from build123d import *

# Parameters (mm, degrees)
SKETCH1_R                = 40
SKETCH1_R_2              = 2.25
BOSS_EXTRUDE1_DEPTH      = 5
SKETCH2_R                = 30
SKETCH2_R_2              = 10
SKETCH2_R_3              = 2.5
BOSS_EXTRUDE2_DEPTH      = 5.5
BOSS_EXTRUDE2_DEPTH_BACK = 10.5
SKETCH3_R                = 2.5
SKETCH3_R_2              = 10
CUT_EXTRUDE1_DEPTH       = 17


with BuildPart() as part:
    # Sketch1 → Boss-Extrude1 (new body)
    with BuildSketch(Plane(origin=(0, 0, 0), x_dir=(1, 0, 0), z_dir=(0, 1, 0))):
        Circle(SKETCH1_R)
        with Locations((0, 35)):
            Circle(SKETCH1_R_2, mode=Mode.SUBTRACT)
        with Locations((30.310889132, 17.5)):
            Circle(SKETCH1_R_2, mode=Mode.SUBTRACT)
        with Locations((30.310889132, -17.5)):
            Circle(SKETCH1_R_2, mode=Mode.SUBTRACT)
        with Locations((0, -35)):
            Circle(SKETCH1_R_2, mode=Mode.SUBTRACT)
        with Locations((-30.310889132, -17.5)):
            Circle(SKETCH1_R_2, mode=Mode.SUBTRACT)
        with Locations((-30.310889132, 17.5)):
            Circle(SKETCH1_R_2, mode=Mode.SUBTRACT)
    extrude(amount=BOSS_EXTRUDE1_DEPTH)

    # Sketch2 → Boss-Extrude2 (add, two sides)
    with BuildSketch(Plane(origin=(0, 5, 0), x_dir=(1, 0, 0), z_dir=(0, 1, 0))) as boss_extrude2_sk:
        Circle(SKETCH2_R)
        Circle(SKETCH2_R_2, mode=Mode.SUBTRACT)
        with Locations((0, -15.25)):
            Circle(SKETCH2_R_3, mode=Mode.SUBTRACT)
        with Locations((-13.206887408, 7.625)):
            Circle(SKETCH2_R_3, mode=Mode.SUBTRACT)
        with Locations((13.206887408, 7.625)):
            Circle(SKETCH2_R_3, mode=Mode.SUBTRACT)
    extrude(amount=BOSS_EXTRUDE2_DEPTH)
    extrude(boss_extrude2_sk.sketch, amount=-BOSS_EXTRUDE2_DEPTH_BACK)

    # Sketch3 → Cut-Extrude1 (cut, through all)
    with BuildSketch(Plane(origin=(0, 10.5, 0), x_dir=(1, 0, 0), z_dir=(0, 1, 0))):
        with Locations((0, -15.25)):
            Circle(SKETCH3_R)
        with Locations((13.206887408, 7.625)):
            Circle(SKETCH3_R)
        Circle(SKETCH3_R_2)
        with Locations((-13.206887408, 7.625)):
            Circle(SKETCH3_R)
    extrude(amount=-CUT_EXTRUDE1_DEPTH, mode=Mode.SUBTRACT)


solid = part.part
Geometry check sheet. Reference: the model listing, model coordinates, mm. A direction names the side the tool comes from. Give positions to 0.01 mm unless a question says otherwise; leave off trailing zeros. Write each loop counter-clockwise with the first axis right and the second up, starting at its lowest first coordinate (ties: lowest second). Pieces come first, ordered by that corner, then holes. Notation, with made-up numbers: M 82.25,-23 L 87.25,-23 A22 cw 87.25,-8 Z; hole C 42.5,37 d5. An arc over 180 degrees is marked long. Answer as CSV lines item,"result". Start each with the question number.
Q1. Section check B-B, the plane z = 0. Record the cut outline in (x, y).
Q2. Section check D-D, the plane y = 2.5. Give the number of separate pieces and of enclosed holes in the cut face, then the cut area to 3 significant figures.
Q3. Material ranges on L1, parallel to Z at x = 0, y = -3.35; L2, parallel to Y at x = 25.5, z = 18.5; L3, parallel to Z at x = 31, y = 3.75, recorded low to high.
Q4. Release check for a two-part mould opening along X. For faces 4 (the face through (6, 5, -30)), 5 (the face through (29.823, 2.465, 19.696)), 6 (the face through (-8.67, 2.46, 39.05)) record: pulls with the +X half, pulls with the -X half, needs draft (parallel to the pull), parting line crosses it, or undercut.
Q5. Section check A-A, the plane x = 0. Record the cut outline in (y, z).
Q6. Section check C-C, the plane z = -17.5. Record the cut outline in (x, y), then the cut area to 3 significant figures.
Q7. Go/stop test with flat-tipped pins: pin 1 (4.5 mm diameter, centred on x = 0, z = 15.25, fed in from -Y); pin 2 (4 mm diameter, centred on y = -1.5, z = -2.5, fed in from +X); pin 3 (6 mm diameter, centred on x = -30.31, z = 17.5, fed in from -Y); pin 4 (6 mm diameter, centred on x = -19, y = 3, fed in from +Z). Record where each tip stops, or that it passes through.
Q8. Tool access check on faces 1 (the face through (-29.97, -2.71, -1.32)), 2 (the face through (-29.97, 7.71, -1.32)), 3 (the face through (13, -5.5, 0)). Record the directions out of +Z, -Z, +X, -X, +Y, -Y that give a thin tool (end or side, any length) a straight path to the whole face; none if there is none.
Geometry says:
1,outline,"M -40,0 L -30,0 L -30,-5.5 L -10,-5.5 L -10,10.5 L -30,10.5 L -30,5 L -40,5 Z; M 10,-5.5 L 30,-5.5 L 30,0 L 40,0 L 40,5 L 30,5 L 30,10.5 L 10,10.5 Z"
2,separate pieces,"1"
2,enclosed holes,"10"
2,area,"4,560 mm^2"
3,L1,"-30 to -10, 10 to 12.75, 17.75 to 30"
3,L2,"0 to 5"
3,L3,"-25.28 to -19.64, -15.36 to 15.36, 19.64 to 25.28"
4,face 4,"needs draft"
4,face 5,"undercut"
4,face 6,"parting line crosses it"
5,outline,"M -5.5,-30 L 0,-30 L 0,-32.75 L 5,-32.75 L 5,-30 L 10.5,-30 L 10.5,-10 L -5.5,-10 Z; M -5.5,10 L 10.5,10 L 10.5,12.75 L -5.5,12.75 Z; M -5.5,17.75 L 10.5,17.75 L 10.5,30 L 5,30 L 5,32.75 L 0,32.75 L 0,30 L -5.5,30 Z; M 0,-40 L 5,-40 L 5,-37.25 L 0,-37.25 Z; M 0,37.25 L 5,37.25 L 5,40 L 0,40 Z"
6,outline,"M -35.97,0 L -32.56,0 L -32.56,5 L -35.97,5 Z; M -28.06,0 L -24.37,0 L -24.37,-5.5 L 24.37,-5.5 L 24.37,0 L 28.06,0 L 28.06,5 L 24.37,5 L 24.37,10.5 L -24.37,10.5 L -24.37,5 L -28.06,5 Z; M 32.56,0 L 35.97,0 L 35.97,5 L 32.56,5 Z"
6,area,"851 mm^2"
7,pin 1,"through"
7,pin 2,"x = 39.98"
7,pin 3,"y = 0"
7,pin 4,"z = 36.66"
8,face 1,"-Y"
8,face 2,"+Y"
8,face 3,"+Z, -Z, +X, -X, -Y"
